Can you work these out from the model? Positions are in its coordinate system, mm. Face numbers are marked on the shaded views. A direction names the side the tool comes from. Round coordinates to 2 decimals unless told otherwise and drop trailing zeros. Write each loop counter-clockwise with the first axis right and the second up, starting at its lowest first coordinate (ties: lowest second). Pieces come first, ordered by that corner, then holes. Notation, with made-up numbers: M 67.25,70.25 L 113.25,70.25 A8 cw 113.25,74.25 Z; hole C 12.25,47 d8. An arc over 180 degrees is marked long. Answer in a Markdown table with one row per item. Add a question column.
(1) Suppose I cut it at B-B, the plane x = 0. Write out the boundary of the cut face in (y, z).
(2) I'm going to push flat-ended pins straight in: pin 1 (2 mm diameter, centred on x = 0.5, y = 0.5, fed in from -Z); pin 2 (0.7 mm diameter, centred on x = 7.5, z = -2, fed in from -Y); pin 3 (2.5 mm diameter, centred on x = -8, z = -2.5, fed in from -Y). Where does each tip first touch, or does it pass through?
(3) If I drill on probe 1 along X at (y, z) = (1, -2.5); probe 2 along X at (y, z) = (-1.25, -1.25); probe 3 along X at (y, z) = (-6, -1.75), over which ranges is the centre line in solid material (lowest first)?
(4) Suppose I cut it at C-C, the plane z = -4.75. Write out the boundary of the cut face in (x, y), then the cut area to 3 significant figures.
(5) For the marked faces 1 and 2, which set-ups out of +Z, -Z, +X, -X, +Y, -Y let a thin tool reach every point of the face, with its end or its side?
(6) If we mould it in two halves opening along X, with no side actions, what happens to the marked faces 3, 4, 5 and 6? For each: released by +X, released by -X, zero draft, split by the parting line, or undercut.
(7) Suppose I cut it at A-A, the plane y = 0. Write out the boundary of the cut face in (x, z), then the cut area to 3 significant figures.
from build123d import *

# Parameters (mm, degrees)
CROQUIS1_R              = 15
SALIENTE_EXTRUIR1_DEPTH = 7
SALIENTE_EXTRUIR1_DRAFT = -13
CROQUIS3_R              = 10
CORTAR_EXTRUIR1_DEPTH   = 3
REDONDEO4_R             = 1
REDONDEO5_R             = 1
CROQUIS4_R              = 2
CORTAR_EXTRUIR3_DEPTH   = 3.5


with BuildPart() as part:
    # Croquis1 → Saliente-Extruir1 (with draft: the straight prism first)
    with BuildSketch(Plane.XY):
        Circle(CROQUIS1_R)
    extrude(amount=-SALIENTE_EXTRUIR1_DEPTH)
    # Saliente-Extruir1: the draft: its side faces are tilted about the plane it starts from
    saliente_extruir1_sides = [part.faces().sort_by_distance(p)[0] for p in [
        (-15, 0, -3.5),
    ]]
    draft(saliente_extruir1_sides, Plane.XY, SALIENTE_EXTRUIR1_DRAFT)

    # Croquis3 → Cortar-Extruir1 (cut)
    with BuildSketch(Plane(origin=(0, 0, -7), x_dir=(-1, 0, 0), z_dir=(0, 0, -1))):
        Circle(CROQUIS3_R)
    extrude(amount=-CORTAR_EXTRUIR1_DEPTH, mode=Mode.SUBTRACT)

    # Redondeo4
    redondeo4_edges = [part.edges().sort_by_distance(p)[0] for p in [
        (10, 0, -7),
    ]]
    fillet(redondeo4_edges, radius=REDONDEO4_R)

    # Redondeo5
    redondeo5_edges = [part.edges().sort_by_distance(p)[0] for p in [
        (-13.383922662, 0, -7),
    ]]
    fillet(redondeo5_edges, radius=REDONDEO5_R)

    # Croquis4 → Cortar-Extruir3 (cut)
    with BuildSketch(Plane(origin=(0, 0, -4), x_dir=(-1, 0, 0), z_dir=(0, 0, -1))):
        with BuildLine():
            Line((6.184658438, 2), (8.5, 2))
            Line((8.5, 2), (8.5, -2))
            Line((8.5, -2), (6.184658438, -2))
            ThreePointArc((6.184658438, -2), (0, -6.5), (-6.184658438, -2))
            Line((-6.184658438, -2), (-8.5, -2))
            Line((-8.5, -2), (-8.5, 2))
            Line((-8.5, 2), (-6.184658438, 2))
            ThreePointArc((-6.184658438, 2), (0, 6.5), (6.184658438, 2))
        make_face()
        Circle(CROQUIS4_R, mode=Mode.SUBTRACT)
    extrude(amount=-CORTAR_EXTRUIR3_DEPTH, mode=Mode.SUBTRACT)


solid = part.part
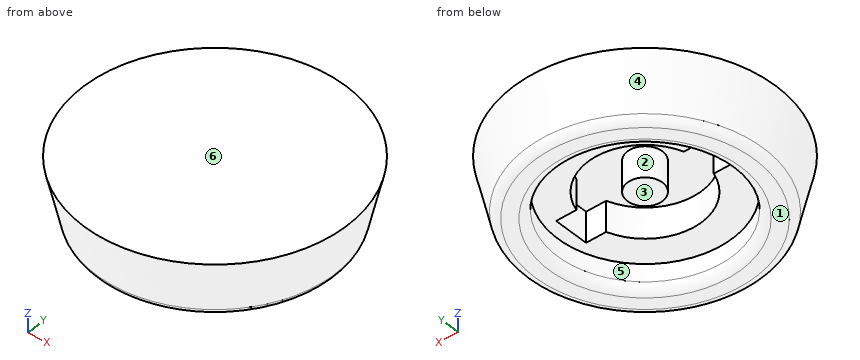
Calculated:
| question | item | result |
|---|---|---|
| 1 | outline | M -15,0 L -13.56,-6.22 A1 ccw -12.59,-7 L -11,-7 A1 ccw -10,-6 L -10,-4 L -6.5,-4 L -6.5,-0.5 L -2,-0.5 L -2,-4 L 2,-4 L 2,-0.5 L 6.5,-0.5 L 6.5,-4 L 10,-4 L 10,-6 A1 ccw 11,-7 L 12.59,-7 A1 ccw 13.56,-6.22 L 15,0 Z |
| 2 | pin 1 | z = -4 |
| 2 | pin 2 | y = -12.68 |
| 2 | pin 3 | y = -12.82 |
| 3 | probe 1 | -14.39 to -8.5, -1.73 to 1.73, 8.5 to 14.39 |
| 3 | probe 2 | -14.66 to -8.5, -1.56 to 1.56, 8.5 to 14.66 |
| 3 | probe 3 | -13.31 to -2.5, 2.5 to 13.31 |
| 4 | outline | C 0,0 d27.81; hole C 0,0 d20 |
| 4 | area | 293 mm² |
| 5 | face 1 | -Z, +X, -X, +Y, -Y |
| 5 | face 2 | -Z |
| 6 | face 3 | undercut |
| 6 | face 4 | split by the parting line |
| 6 | face 5 | undercut |
| 6 | face 6 | zero draft |
| 7 | outline | M -15,0 L -13.56,-6.22 A1 ccw -12.59,-7 L -11,-7 A1 ccw -10,-6 L -10,-4 L -8.5,-4 L -8.5,-0.5 L -2,-0.5 L -2,-4 L 2,-4 L 2,-0.5 L 8.5,-0.5 L 8.5,-4 L 10,-4 L 10,-6 A1 ccw 11,-7 L 12.59,-7 A1 ccw 13.56,-6.22 L 15,0 Z |
| 7 | area | 92.5 mm² |
